Work out the finished part from the listing and answer in its coordinate system (mm). A direction names the side the tool comes from. Round coordinates to 2 decimals unless told otherwise and drop trailing zeros. Write each loop counter-clockwise with the first axis right and the second up, starting at its lowest first coordinate (ties: lowest second). Pieces come first, ordered by that corner, then holes. Notation, with made-up numbers: M -22.5,-35 L -5.5,-35 A6 cw -5.5,-24 Z; hole C 26.5,28 d2. An arc over 180 degrees is marked long. One line per item, written item: value. Start each with the question number.
Q1. Find section C-C (y = 13.5). Write down the section's boundary in (x, z), and give its area (3 significant figures).
Q2. Given pin 1 Ø12 at (y, z) = (7, -24) entering from -X; pin 2 Ø21.5 at (x, z) = (-5, -9) entering from +Y; pin 3 Ø1 at (x, z) = (30.5, -28.5) entering from -Y; pin 4 Ø12 at (x, y) = (-44.5, 33.5) entering from +Z, each flat-ended and moving along its own axis, determine where each tip first touches the part or whether it passes through.
Q3. Find section D-D (z = 10.5). Write down the section's boundary in (x, y), and give its area (3 significant figures).
Q4. Find section B-B (z = -1). Write down the section's boundary in (x, y), and give its area (3 significant figures).
Q5. The mould has two halves that part along X. Classify faces 1 (the cylindrical face through (0.66, 4.93, -14.985)), 2 (the flat face through (41.989, 24.65, -31.183)), 3 (the flat face through (-43, 24.6, -30.6)): released by +X, released by -X, zero draft, split by the parting line, or undercut.
Q6. Find section A-A (x = 0). Write down the section's boundary in (y, z), and give its area (4 significant figures).
Q7. Consider probe 1 along X at (y, z) = (6, 0); probe 2 along Y at (x, z) = (22.5, -20); probe 3 along Z at (x, y) = (4, 7). Determine where each line is inside the solid, lowest interval first.
Q8. A tool of negligible diameter and unlimited length cuts with its end or side. For faces 4 (the flat face through (-1, 10, -18)), 5 (the flat face through (6, 50, -43)), from which of +Z, -Z, +X, -X, +Y, -Y can it reach the whole face along a straight path? Write none if from no direction.
from build123d import *

# Parameters (mm, degrees)
RESSALTO_EXTRUS_O4_DEPTH = 50
ESBO_O1_7_R              = 15
RESSALTO_EXTRUS_O5_DEPTH = 10
CORTE_EXTRUS_O1_REACH    = 128.396
ESBO_O2_R                = 7.5
CORTE_EXTRUS_O2_REACH    = 128.396
ESBO_O3_R                = 7.5


with BuildPart() as part:
    # Esbo_o1 → Ressalto-extrus_o4 (new body)
    with BuildSketch(Plane(origin=(0, 0, 0), x_dir=(1, 0, 0), z_dir=(0, 1, 0))):
        with BuildLine():
            Line((-2, 45.033320997), (-75, 2.886751346))
            Line((-75, 2.886751346), (-79, 9.814954576))
            Line((-79, 9.814954576), (-6, 51.961524227))
            ThreePointArc((-6, 51.961524227), (0, 53.569219382), (6, 51.961524227))
            Line((6, 51.961524227), (79, 9.814954576))
            Line((79, 9.814954576), (75, 2.886751346))
            Line((75, 2.886751346), (2, 45.033320997))
            ThreePointArc((2, 45.033320997), (0, 45.569219382), (-2, 45.033320997))
        make_face()
    extrude(amount=RESSALTO_EXTRUS_O4_DEPTH)

    # Esbo_o1_7 → Ressalto-extrus_o5 (add)
    with BuildSketch(Plane(origin=(0, 0, 0), x_dir=(1, 0, 0), z_dir=(0, 1, 0))):
        with BuildLine():
            ThreePointArc((2, 45.033320997), (0, 45.569219382), (-2, 45.033320997))
            Line((-2, 45.033320997), (-75, 2.886751346))
            Line((-75, 2.886751346), (-25, -25.980762114))
            Line((-25, -25.980762114), (25, -25.980762114))
            Line((25, -25.980762114), (75, 2.886751346))
            Line((75, 2.886751346), (2, 45.033320997))
        make_face()
        with Locations(Location((0, 0, 0), (0, 0, 270))):
            Circle(ESBO_O1_7_R, mode=Mode.SUBTRACT)
    extrude(amount=RESSALTO_EXTRUS_O5_DEPTH)

    # Esbo_o2 → Corte-extrus_o1 (cut, up to next)
    with BuildSketch(Plane(origin=(-20, 0, -34.641016151), x_dir=(0.866025403784438, 0, -0.5000000000000012), z_dir=(0.5000000000000011, 0, 0.8660254037844379)), mode=Mode.PRIVATE) as corte_extrus_o1_sk1:
        with Locations((-33.508529611, 30)):
            Circle(ESBO_O2_R)
    corte_extrus_o1_tool1 = extrude(corte_extrus_o1_sk1.sketch, amount=-CORTE_EXTRUS_O1_REACH, mode=Mode.PRIVATE) & part.part
    add(corte_extrus_o1_tool1.solids().sort_by_distance((-49.019238, 30, -17.886751))[0], mode=Mode.SUBTRACT)

    # Esbo_o3 → Corte-extrus_o2 (cut, up to next)
    with BuildSketch(Plane(origin=(20, 0, -34.641016151), x_dir=(0.866025403784438, 0, 0.5000000000000012), z_dir=(-0.5000000000000011, 0, 0.8660254037844379)), mode=Mode.PRIVATE) as corte_extrus_o2_sk1:
        with Locations((33.508529611, 30)):
            Circle(ESBO_O3_R)
    corte_extrus_o2_tool1 = extrude(corte_extrus_o2_sk1.sketch, amount=-CORTE_EXTRUS_O2_REACH, mode=Mode.PRIVATE) & part.part
    add(corte_extrus_o2_tool1.solids().sort_by_distance((49.019238, 30, -17.886751))[0], mode=Mode.SUBTRACT)


solid = part.part
The answers:
1. outline: M -79,-9.81 L -6,-51.96 A12 ccw 6,-51.96 L 79,-9.81 L 75,-2.89 L 2,-45.03 A4 cw -2,-45.03 L -75,-2.89 Z
1. area: 1,420 mm2
2. pin 1: x = -64.82
2. pin 2: y = 10
2. pin 3: y = 0
2. pin 4: z = -17.91
3. outline: M -51.81,0 L -10.71,0 L -10.71,10 L -51.81,10 Z; M 10.71,0 L 51.81,0 L 51.81,10 L 10.71,10 Z
3. area: 822 mm2
4. outline: M -71.73,0 L -14.97,0 L -14.97,10 L -71.73,10 Z; M 14.97,0 L 71.73,0 L 71.73,10 L 14.97,10 Z
4. area: 1,140 mm2
5. face 1: undercut
5. face 2: released by +X
5. face 3: released by -X
6. outline: M 0,-53.57 L 50,-53.57 L 50,-45.57 L 10,-45.57 L 10,-15 L 0,-15 Z; M 0,15 L 10,15 L 10,25.98 L 0,25.98 Z
6. area: 815.5 mm2
7. probe 1: -70 to -15, 15 to 70
7. probe 2: 0 to 10
7. probe 3: -52.88 to -14.46, 14.46 to 25.98
8. face 4: +Z, +Y
8. face 5: +Z, -Z, +X, -X, +Y
